Can you work these out from the model? Positions are in its coordinate system, mm. Face numbers are marked on the shaded views. A direction names the side the tool comes from. Coordinates: 2 decimals unless noted, no trailing zeros. Write each loop counter-clockwise with the first axis right and the second up, starting at its lowest first coordinate (ties: lowest second). Pieces come first, ordered by that corner, then holes. Notation, with made-up numbers: (34.25, -15) - (73.25, -15) arc R5 cw to (73.25, -6) - close; hole circle Ø1 at (75, -30.75). An arc over 180 degrees is marked (long way). Use one line per item in the form item = value. Start each with the question number.
(1) If I drill on probe 1 along X at (y, z) = (-196.5, 0); probe 2 along Z at (x, y) = (19, -196); probe 3 along X at (y, z) = (93, 19), over which ranges is the centre line in solid material (lowest first)? Write a range as from..to.
(2) If we section it at C-C on y = -101: Please give me the cut outline in (x, z), then the cut area to 3 significant figures.
(3) If we section it at A-A on z = 0: Please give me the cut outline in (x, y), then the cut area to 3 significant figures.
(4) For pin 1 Ø8 at (x, y) = (22, -24) entering from +Z; pin 2 Ø7.5 at (x, z) = (-10.4, 0) entering from -Y; pin 3 Ø12 at (y, z) = (-86, 1.5) entering from +X, each with a flat end and sliding along its axis, tell me the tip position at first contact or that it passes through.
(5) On a 3-axis mill with a long thin cutter (end or side, diameter ignored), from which of +Z, -Z, +X, -X, +Y, -Y can I reach the whole of each face in a straight line? I mean the marked faces 1 and 2. Say none if no direction works.
(6) If we section it at B-B on x = -10.4: Please give me the cut outline in (y, z).
```python
from build123d import *

# Parameters (mm, degrees)
SKETCH1_W           = 60
SKETCH1_H           = 50
BOSS_EXTRUDE1_DEPTH = 200
SKETCH2_W           = 40
SKETCH2_H           = 390
CUT_EXTRUDE1_DEPTH  = 50
SKETCH4_R           = 4.2
CUT_EXTRUDE3_DEPTH  = 402.901729282


with BuildPart() as part:
    # Sketch1 → Boss-Extrude1 (new, symmetric)
    with BuildSketch(Plane(origin=(0, 0, 0), x_dir=(1, 0, 0), z_dir=(0, 1, 0))):
        Rectangle(SKETCH1_W, SKETCH1_H)
    extrude(amount=BOSS_EXTRUDE1_DEPTH, both=True)

    # Sketch2 → Cut-Extrude1 (cut)
    with BuildSketch(Plane(origin=(30, 0, 0), x_dir=(0, 0, -1), z_dir=(1, 0, 0))):
        with Locations((-5, 5)):
            Rectangle(SKETCH2_W, SKETCH2_H)
    extrude(amount=-CUT_EXTRUDE1_DEPTH, mode=Mode.SUBTRACT)

    # Sketch4 → Cut-Extrude3 (cut, through all)
    with BuildSketch(Plane.XZ.offset(200)):
        with Locations(Location((-10.4, 0, 0), (0, 0, 270))):
            Circle(SKETCH4_R)
        with Locations(Location((19.6, 0, 0), (0, 0, 270))):
            Circle(SKETCH4_R)
    extrude(amount=-CUT_EXTRUDE3_DEPTH, mode=Mode.SUBTRACT)


solid = part.part
```
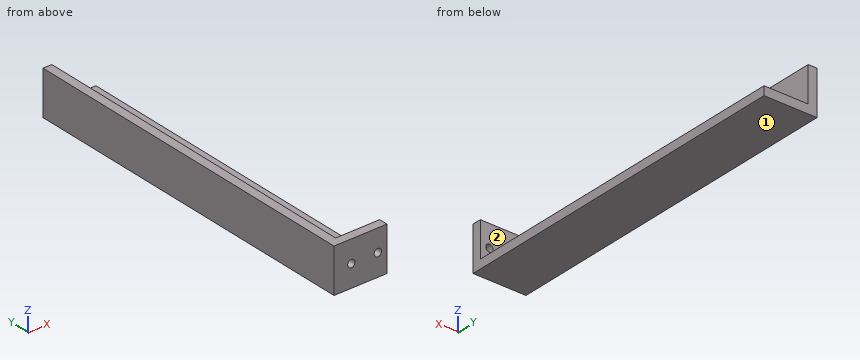
Reported:
q1.probe_1 = -30..-14.6, -6.2..15.4, 23.8..30
q1.probe_2 = -25..-4.16, 4.16..25
q1.probe_3 = -30..-20
q2.outline = (-30, -25) - (30, -25) - (30, -15) - (-20, -15) - (-20, 25) - (-30, 25) - close
q2.area = 1,000 mm2
q3.outline = (-30, -200) - (-14.6, -200) - (-14.6, -190) - (-20, -190) - (-20, 200) - (-30, 200) - close; (-6.2, -200) - (15.4, -200) - (15.4, -190) - (-6.2, -190) - close; (23.8, -200) - (30, -200) - (30, -190) - (23.8, -190) - close
q3.area = 4,330 mm2
q4.pin_1 = -15
q4.pin_2 = through
q4.pin_3 = -20
q5.face_1 = -Z, +X, -X, +Y, -Y
q5.face_2 = +Z, +X, +Y
q6.outline = (-200, -25) - (200, -25) - (200, -15) - (-190, -15) - (-190, -4.2) - (-200, -4.2) - close; (-200, 4.2) - (-190, 4.2) - (-190, 25) - (-200, 25) - close
